```python
from build123d import *

# Parameters (mm, degrees)
F0_W     = 740
F0_H     = 36
F1_DEPTH = 9
F2_SIZE  = 35.99999
F4_DEPTH = 9


# Not quite as in the source:
# - a fillet or chamfer is up to 0.001 mm smaller than in the source, because OpenCascade refuses the exact size


with BuildPart() as f1:
    # F0 (on Top) → F1 (new body)
    with BuildSketch(Plane.XY):
        Rectangle(F0_W, F0_H)
    extrude(amount=F1_DEPTH)

    # F2 (size 36 in the source; OpenCascade refuses exactly that, so slightly less here)
    f2_edges = [f1.edges().sort_by_distance(p)[0] for p in [
        (-370, -18, 4.5),
        (370, -18, 4.5),
    ]]
    chamfer(f2_edges, length=F2_SIZE)

    # F3 (on face) → F4 (cut, through all)
    with BuildSketch(Plane.XY.offset(9)):
        Polygon((-301.5692193817, -18), (-68.4307806183, -18), (-110, 6), (-260, 6), align=None)
    extrude(amount=-F4_DEPTH, mode=Mode.SUBTRACT)


solid = f1.part
```
Model file for the job. Use its own axes, mm. Give positions to 0.01 mm unless a question says otherwise; leave off trailing zeros. Loops run counter-clockwise (first coordinate to the right, second up) from the corner with the lowest first, then second, coordinate; pieces in that order, holes last. Notation, with made-up numbers: (63, 58) - (104, 58) arc R3 cw to (104, 63) - close; hole circle Ø1 at (1.25, 84). An arc over 180 degrees is marked (long way). One line per item, written item: value. Start each with the question number.
1. Pull direction X, two halves, no side cores. Call faces 1 (the flat face through (-5, 0, 9)), 2 (the flat face through (-88.92, -6.17, 4.56)), 3 (the flat face through (-280.49, -5.83, 4.56)), 4 (the flat face through (352, 0, 4)): pulls with the +X half, pulls with the -X half, needs draft (parallel to the pull), parting line crosses it, or undercut.
2. Probe L1, parallel to Y at x = -156, z = 1.5; L2, parallel to X at y = 0.5, z = 4; L3, parallel to X at y = 0, z = 5.5. List the from-to ranges inside material, lowest first. Write a range as from..to.
3. Slice it at A-A (y = -7.5). List the corners of the cut face in (x, z), plus the area to 3 significant figures.
4. Pin check, flat tip, straight feed: pin 1 (2 mm diameter, centred on y = 7, z = 6.5, fed in from -X). Stop position of the tip, or through.
5. Slice it at C-C (x = -86.5). List the corners of the cut face in (y, z), plus the area to 3 significant figures.
Solution:
1. face 1: needs draft
1. face 2: undercut
1. face 3: undercut
1. face 4: pulls with the +X half
2. L1: y = 6..18
2. L2: x = -352.5..-269.53, -100.47..352.5
2. L3: x = -352..-270.39, -99.61..352
3. outline: (-344.5, 0) - (-283.38, 0) - (-283.38, 9) - (-344.5, 9) - close; (-86.62, 0) - (344.5, 0) - (344.5, 9) - (-86.62, 9) - close
3. area: 4,430 mm^2
4. pin 1: stops at x = -360
5. outline: (-7.57, 0) - (18, 0) - (18, 9) - (-7.57, 9) - close
5. area: 230 mm^2
